from build123d import *

# Parameters (mm, degrees)
SKETCH1_R                   = 50.8
BOSS_EXTRUDE1_DEPTH         = 2.9718
SKETCH2_R                   = 2.54
CUT_EXTRUDE1_DEPTH          = 73.087491155
CIRPATTERN1_COUNT           = 6
CUT_EXTRUDE2_DEPTH          = 73.087491155
F_32_0_116_DIAMETER_HOLE1_D = 2.9464
CIRPATTERN2_COUNT           = 3


with BuildPart() as part:
    # Sketch1 → Boss-Extrude1 (new, symmetric)
    with BuildSketch(Plane.XY):
        Circle(SKETCH1_R)
    extrude(amount=BOSS_EXTRUDE1_DEPTH, both=True)

    # Sketch2 → Cut-Extrude1 (cut, through all)
    with BuildSketch(Plane.XY.offset(2.9718)):
        with Locations((0, 44.45)):
            Circle(SKETCH2_R)
    cut_extrude1 = extrude(amount=-CUT_EXTRUDE1_DEPTH, mode=Mode.SUBTRACT)

    # CirPattern1: Cut-Extrude1 ×6 about axis
    cirpattern1_axis = Axis((0, 0, 0), (0, 0, 1))
    for i in range(1, CIRPATTERN1_COUNT):
        add(cut_extrude1.rotate(cirpattern1_axis, i * 360 / CIRPATTERN1_COUNT), mode=Mode.SUBTRACT)

    # Sketch3 → Cut-Extrude2 (cut, through all)
    with BuildSketch(Plane.XY.offset(2.9718)):
        Polygon((0, 3.519527241), (3.048, 1.75976362), (3.048, -1.75976362), (0, -3.519527241), (-3.048, -1.75976362), (-3.048, 1.75976362), align=None)
    extrude(amount=-CUT_EXTRUDE2_DEPTH, mode=Mode.SUBTRACT)

    # 32 _0.116_ Diameter Hole1 (through all)
    with Locations(Plane.XY.offset(2.9718)):
        with Locations((0, 15.24)):
            f_32_0_116_diameter_hole1 = Hole(F_32_0_116_DIAMETER_HOLE1_D / 2)

    # CirPattern2: 32 _0.116_ Diameter Hole1 ×3 about axis
    cirpattern2_axis = Axis((0, 0, 0), (0, 0, 1))
    for i in range(1, CIRPATTERN2_COUNT):
        add(f_32_0_116_diameter_hole1.rotate(cirpattern2_axis, i * 360 / CIRPATTERN2_COUNT), mode=Mode.SUBTRACT)


solid = part.part
Design review of the part built by this model. Coordinates are the model's own, in mm. A direction names the side the tool comes from. Round coordinates to 2 decimals unless told otherwise and drop trailing zeros. Write each loop counter-clockwise with the first axis right and the second up, starting at its lowest first coordinate (ties: lowest second). Pieces come first, ordered by that corner, then holes.
Item 1: Consider section A-A on y = 0. Give the boundary of the cut face in (x, z), and give its area (3 significant figures).
Item 2: Consider section B-B on z = -1.9. Count the separate pieces of the cut face and the enclosed holes in it, and give its area (3 significant figures).
Item 3: Consider section D-D on x = -31. Give the boundary of the cut face in (y, z), and give its area (3 significant figures).
Item 4: For faces 4 (the flat face through (-3.048, 0, 0)), 5 (the flat face through (11, 1, -2.972)), list the 3-axis set-ups (+Z, -Z, +X, -X, +Y, -Y) from which the entire face can be reached by the end or side of a thin tool; tool diameter is ignored.
Item 5: For pin 1 Ø2 at (x, z) = (-23, 0) entering from -Y; pin 2 Ø4.5 at (x, y) = (-38.49, -22.22) entering from +Z; pin 3 Ø1 at (x, z) = (-27, -2) entering from -Y; pin 4 Ø3 at (y, z) = (-3.5, -1) entering from +X, all flat-tipped, find the tip position at first contact; note any pin that passes through.
Item 6: Draft analysis for pull direction X (two halves, no side actions). For faces 1 (the flat face through (11, 1, 2.972)), 2 (the cylindrical face through (-11.012, -49.592, 0.042)), 3 (the flat face through (-1.503, -2.652, 0.042)), state which applies: released by +X, released by -X, zero draft, split by the parting line, or undercut.
Item 7: Consider section C-C on y = 44.45. Give the boundary of the cut face in (x, z), and give its area (3 significant figures).
Item 8: Wall thickness on L1, parallel to X at y = -20.5, z = -0.7; L2, parallel to Y at x = 2, z = 2.55; L3, parallel to X at y = 21.5, z = -1.9: over which ranges is each line inside the solid? List them lowest first.
Check values:
1. outline: (-50.8, -2.97) - (-3.05, -2.97) - (-3.05, 2.97) - (-50.8, 2.97) - close; (3.05, -2.97) - (50.8, -2.97) - (50.8, 2.97) - (3.05, 2.97) - close
1. area: 568 mm2
2. separate pieces: 1
2. enclosed holes: 10
2. area: 7,930 mm2
3. outline: (-40.24, -2.97) - (40.24, -2.97) - (40.24, 2.97) - (-40.24, 2.97) - close
3. area: 478 mm2
4. face 4: +Z, -Z
4. face 5: -Z, +X, -X, +Y, -Y
5. pin 1: stops at y = -45.79
5. pin 2: passes through
5. pin 3: stops at y = -43.34
5. pin 4: stops at x = 50.76
6. face 1: zero draft
6. face 2: split by the parting line
6. face 3: undercut
7. outline: (-24.59, -2.97) - (-2.54, -2.97) - (-2.54, 2.97) - (-24.59, 2.97) - close; (2.54, -2.97) - (24.59, -2.97) - (24.59, 2.97) - (2.54, 2.97) - close
7. area: 262 mm2
8. L1: x = -46.48 to -40.36, -36.63 to 36.63, 40.36 to 46.48
8. L2: y = -50.76 to -46.02, -42.88 to -2.36, 2.36 to 42.88, 46.02 to 50.76
8. L3: x = -46.03 to -40.93, -36.06 to 36.06, 40.93 to 46.03
